```python
from build123d import *

# Parameters (mm, degrees)
ESQUISSE1_R        = 12.5
BOSS_EXTRU_1_DEPTH = 54.5
ESQUISSE2_R        = 1.5
BOSS_EXTRU_2_DEPTH = 7
ESQUISSE3_R        = 16
BOSS_EXTRU_3_DEPTH = 39.85
ESQUISSE4_R        = 10
BOSS_EXTRU_4_DEPTH = 3
ESQUISSE5_R        = 3
BOSS_EXTRU_5_DEPTH = 17
ESQUISSE6_R        = 1.5
BOSS_EXTRU_6_DEPTH = 15


with BuildPart() as part:
    # Esquisse1 → Boss.-Extru.1 (new body)
    with BuildSketch(Plane.XY):
        Circle(ESQUISSE1_R)
    extrude(amount=BOSS_EXTRU_1_DEPTH)

    # Esquisse2 → Boss.-Extru.2 (add)
    with BuildSketch(Plane.XY.offset(54.5)):
        Circle(ESQUISSE2_R)
    extrude(amount=BOSS_EXTRU_2_DEPTH)

    # Esquisse3 → Boss.-Extru.3 (add)
    with BuildSketch(Plane(origin=(0, 0, 0), x_dir=(-1, 0, 0), z_dir=(0, 0, -1))):
        Circle(ESQUISSE3_R)
    extrude(amount=BOSS_EXTRU_3_DEPTH)

    # Esquisse4 → Boss.-Extru.4 (add)
    with BuildSketch(Plane(origin=(0, 0, -39.85), x_dir=(-1, 0, 0), z_dir=(0, 0, -1))):
        Circle(ESQUISSE4_R)
    extrude(amount=BOSS_EXTRU_4_DEPTH)

    # Esquisse5 → Boss.-Extru.5 (add)
    with BuildSketch(Plane(origin=(0, 0, -42.85), x_dir=(-1, 0, 0), z_dir=(0, 0, -1))):
        Circle(ESQUISSE5_R)
    extrude(amount=BOSS_EXTRU_5_DEPTH)

    # Esquisse6 → Boss.-Extru.6 (add)
    with BuildSketch(Plane.XY.offset(54.5)):
        with Locations((0, 10)):
            Circle(ESQUISSE6_R)
        with Locations((0, -10)):
            Circle(ESQUISSE6_R)
    extrude(amount=BOSS_EXTRU_6_DEPTH)


solid = part.part
```
CAD build for the part. Positions are in the model's coordinates, mm. A direction names the side the tool comes from. Give positions to 0.01 mm unless a question says otherwise; leave off trailing zeros. Order: outer loops, then holes, each group sorted by start corner. A loop starts at its lowest first (then second) coordinate and runs counter-clockwise, first axis right, second up.
(1) Saw through at C-C, the plane z = 6. Give the cut face in (x, y).
(2) Saw through at A-A, the plane x = 0. Give the cut face in (y, z).
(3) Saw through at B-B, the plane y = 0. Give the cut face in (x, z), then the cut area to 3 significant figures.
(4) Mould opens along Y. For faces 6 (the cylindrical face through (2.17, -9.76, -41.33)), 7 (the cylindrical face through (-1.5, 0.07, 57.95)), 8 (the flat face through (0, 0, -59.85)) say: released by +Y, released by -Y, zero draft, split by the parting line, or undercut.
(5) Flat gauge pins, fed straight in: pin 1 (9.5 mm diameter, centred on x = 6.5, y = 3, fed in from +Z); pin 2 (6 mm diameter, centred on x = 3, z = -44, fed in from +Y); pin 3 (1.5 mm diameter, centred on x = 0.5, y = -0.5, fed in from +Z); pin 4 (10 mm diameter, centred on y = -0.5, z = -19, fed in from -X). Where does each tip first touch, or does it go through?
(6) Drill centre lines: L1, parallel to Z at x = -8, y = 5; L2, parallel to Z at x = -7, y = 8; L3, parallel to Y at x = -12.5, z = -30. Where is each one in solid material? Low to high.
(7) Tool access for faces 1 (the flat face through (0, -10, 69.5)), 2 (the flat face through (-2.1, 2.4, -42.85)), 3 (the flat face through (10, -8, 0)), 4 (the flat face through (0, 0, 61.5)), 5 (the cylindrical face through (3.47, -15.62, -19.65)): list every direction of +Z, -Z, +X, -X, +Y, -Y with a clear straight run to the whole face (end or side of a thin tool).
(8) Saw through at D-D, the plane y = -7. Give the cut face in (x, z).
Results found:
1. outline: circle Ø25 at (0, 0)
2. outline: (-16, -39.85) - (-10, -39.85) - (-10, -42.85) - (-3, -42.85) - (-3, -59.85) - (3, -59.85) - (3, -42.85) - (10, -42.85) - (10, -39.85) - (16, -39.85) - (16, 0) - (12.5, 0) - (12.5, 54.5) - (11.5, 54.5) - (11.5, 69.5) - (8.5, 69.5) - (8.5, 54.5) - (1.5, 54.5) - (1.5, 61.5) - (-1.5, 61.5) - (-1.5, 54.5) - (-8.5, 54.5) - (-8.5, 69.5) - (-11.5, 69.5) - (-11.5, 54.5) - (-12.5, 54.5) - (-12.5, 0) - (-16, 0) - close
3. outline: (-16, -39.85) - (-10, -39.85) - (-10, -42.85) - (-3, -42.85) - (-3, -59.85) - (3, -59.85) - (3, -42.85) - (10, -42.85) - (10, -39.85) - (16, -39.85) - (16, 0) - (12.5, 0) - (12.5, 54.5) - (1.5, 54.5) - (1.5, 61.5) - (-1.5, 61.5) - (-1.5, 54.5) - (-12.5, 54.5) - (-12.5, 0) - (-16, 0) - close
3. area: 2,820 mm2
4. face 6: split by the parting line
4. face 7: undercut
4. face 8: zero draft
5. pin 1: stops at z = 54.5
5. pin 2: stops at y = 10
5. pin 3: stops at z = 61.5
5. pin 4: stops at x = -16
6. L1: z = -42.85 to 54.5
6. L2: z = -39.85 to 54.5
6. L3: y = -9.99 to 9.99
7. face 1: +Z, +X, -X, +Y, -Y
7. face 2: -Z
7. face 3: +Z
7. face 4: +Z, +X, -X
7. face 5: +Z, -Z
8. outline: (-14.39, -39.85) - (-7.14, -39.85) - (-7.14, -42.85) - (7.14, -42.85) - (7.14, -39.85) - (14.39, -39.85) - (14.39, 0) - (10.36, 0) - (10.36, 54.5) - (-10.36, 54.5) - (-10.36, 0) - (-14.39, 0) - close
